from build123d import *

# Parameters (mm, degrees)
ESQUISSE1_W             = 34
ESQUISSE1_H             = 100.65
BOSS_EXTRU_1_DEPTH      = 12.5
ESQUISSE2_W             = 31
ESQUISSE2_H             = 97.65
ENL_V_MAT_EXTRU_1_DEPTH = 11
ESQUISSE5_R             = 2
BOSS_EXTRU_4_DEPTH      = 3
CONG_2_R                = 2
CONG_3_R                = 2
CONG_4_R                = 2
ESQUISSE7_W             = 7.5
ESQUISSE7_H             = 80
BOSS_EXTRU_6_DEPTH      = 1
ESQUISSE9_W             = 9.45
ESQUISSE9_H             = 80
BOSS_EXTRU_7_DEPTH      = 1.7
ESQUISSE11_W            = 15.5
ESQUISSE11_H            = 4.6
ENL_V_MAT_EXTRU_3_DEPTH = 3
CONG_7_R                = 1
ESQUISSE12_R            = 1.3
ENL_V_MAT_EXTRU_5_DEPTH = 3


with BuildPart() as part:
    # Esquisse1 → Boss.-Extru.1 (new body)
    with BuildSketch(Plane.XY):
        with Locations((17, 50.325)):
            Rectangle(ESQUISSE1_W, ESQUISSE1_H)
    extrude(amount=BOSS_EXTRU_1_DEPTH)

    # Esquisse2 → Enlèv. mat.-Extru.1 (cut)
    with BuildSketch(Plane.XY.offset(12.5)):
        with Locations((17, 50.325)):
            Rectangle(ESQUISSE2_W, ESQUISSE2_H)
    extrude(amount=-ENL_V_MAT_EXTRU_1_DEPTH, mode=Mode.SUBTRACT)

    # Esquisse5 → Boss.-Extru.4 (add)
    with BuildSketch(Plane.XY.offset(1.5)):
        with Locations((5.5, 63.5)):
            Circle(ESQUISSE5_R)
        with Locations((28.5, 63.5)):
            Circle(ESQUISSE5_R)
        with Locations((5.5, 5.5)):
            Circle(ESQUISSE5_R)
        with Locations((28.5, 5.5)):
            Circle(ESQUISSE5_R)
    extrude(amount=BOSS_EXTRU_4_DEPTH)

    # Congé2
    cong_2_edges = [part.edges().sort_by_distance(p)[0] for p in [
        (34, 0, 6.25),
    ]]
    fillet(cong_2_edges, radius=CONG_2_R)

    # Congé3
    cong_3_edges = [part.edges().sort_by_distance(p)[0] for p in [
        (34, 100.65, 6.25),
    ]]
    fillet(cong_3_edges, radius=CONG_3_R)

    # Congé4
    cong_4_edges = [part.edges().sort_by_distance(p)[0] for p in [
        (34, 50.325, 0),
        (33.414213562, 0.585786438, 0),
        (16, 100.65, 0),
        (33.414213562, 100.064213562, 0),
        (16, 0, 0),
    ]]
    fillet(cong_4_edges, radius=CONG_4_R)

    # Esquisse7 → Boss.-Extru.6 (add)
    with BuildSketch(Plane.ZY):
        with Locations((7, 55.45)):
            Rectangle(ESQUISSE7_W, ESQUISSE7_H)
    extrude(amount=BOSS_EXTRU_6_DEPTH)

    # Esquisse9 → Boss.-Extru.7 (add)
    with BuildSketch(Plane.ZY.offset(1)):
        with Locations((6.725, 55.45)):
            Rectangle(ESQUISSE9_W, ESQUISSE9_H)
    extrude(amount=BOSS_EXTRU_7_DEPTH)

    # Esquisse11 → Enlèv. mat.-Extru.3 (cut)
    with BuildSketch(Plane(origin=(0, 1.5, 0), x_dir=(1, 0, 0), z_dir=(0, 1, 0))):
        with Locations((14.724178104, -7.8)):
            Rectangle(ESQUISSE11_W, ESQUISSE11_H)
    extrude(amount=-ENL_V_MAT_EXTRU_3_DEPTH, mode=Mode.SUBTRACT)

    # Congé7
    cong_7_edges = [part.edges().sort_by_distance(p)[0] for p in [
        (-2.7, 55.45, 2),
        (-2.7, 15.45, 6.725),
        (-2.7, 55.45, 11.45),
        (-2.7, 95.45, 6.725),
    ]]
    fillet(cong_7_edges, radius=CONG_7_R)

    # Esquisse12 → Enlèv. mat.-Extru.5 (cut)
    with BuildSketch(Plane.XY.offset(4.5)):
        with Locations((5.5, 63.5)):
            Circle(ESQUISSE12_R)
        with Locations((28.5, 63.5)):
            Circle(ESQUISSE12_R)
        with Locations((5.5, 5.5)):
            Circle(ESQUISSE12_R)
        with Locations((28.5, 5.5)):
            Circle(ESQUISSE12_R)
    extrude(amount=-ENL_V_MAT_EXTRU_5_DEPTH, mode=Mode.SUBTRACT)


solid = part.part
Geometry check sheet. Reference: the model listing, model coordinates, mm. A direction names the side the tool comes from. Give positions to 0.01 mm unless a question says otherwise; leave off trailing zeros. Write each loop counter-clockwise with the first axis right and the second up, starting at its lowest first coordinate (ties: lowest second). Pieces come first, ordered by that corner, then holes. Notation, with made-up numbers: (65.5, 87.5) - (99.5, 87.5) arc R27 cw to (99.5, 110.5) - close; hole circle Ø3 at (-36, 52.25). An arc over 180 degrees is marked (long way). Put each result on its own line as item: value.
1. Set-up check for faces 1 (the flat face through (-1, 95.45, 7)), 2 (the flat face through (34, 50, 7)), 3 (the flat face through (5, 6, 1.5)): record each of +Z, -Z, +X, -X, +Y, -Y from which the full face is reachable in a straight line by a thin tool's end or side.
Ans:
face 1: +Z, -Z, -X, +Y
face 2: +Z, -Z, +X, +Y, -Y
face 3: +Z
2. Sectioned sample at A-A, the plane x = 15.5. Enter the section's corners in (y, z), plus the area to 3 significant figures.
Ans:
outline: (0, 2) arc R2 ccw to (2, 0) - (98.65, 0) arc R2 ccw to (100.65, 2) - (100.65, 12.5) - (99.15, 12.5) - (99.15, 1.5) - (1.5, 1.5) - (1.5, 5.5) - (0, 5.5) - close; (0, 10.1) - (1.5, 10.1) - (1.5, 12.5) - (0, 12.5) - close
area: 175 mm²
3. Draft check along Y on faces 4 (the flat face through (16, 0, 5)), 5 (the cylindrical face through (33.4, 51, 0.57)), 6 (the flat face through (1.5, 50, 7)). Enter one of: +Y half, -Y half, draft (parallel to the pull), parting line (faces both ways), or undercut.
Ans:
face 4: -Y half
face 5: draft
face 6: undercut
4. Sectioned sample at D-D, the plane x = 5.5. Enter the section's corners in (y, z).
Ans:
outline: (0, 2) arc R2 ccw to (2, 0) - (98.65, 0) arc R2 ccw to (100.65, 2) - (100.65, 12.5) - (99.15, 12.5) - (99.15, 1.5) - (65.5, 1.5) - (65.5, 4.5) - (64.8, 4.5) - (64.8, 1.5) - (62.2, 1.5) - (62.2, 4.5) - (61.5, 4.5) - (61.5, 1.5) - (7.5, 1.5) - (7.5, 4.5) - (6.8, 4.5) - (6.8, 1.5) - (4.2, 1.5) - (4.2, 4.5) - (3.5, 4.5) - (3.5, 1.5) - (1.5, 1.5) - (1.5, 12.5) - (0, 12.5) - close
5. Sectioned sample at C-C, the plane z = 8. Enter the section's corners in (x, y), plus the area to 3 significant figures.
Ans:
outline: (-2.7, 16.45) arc R1 ccw to (-1.7, 15.45) - (0, 15.45) - (0, 0) - (6.97, 0) - (6.97, 1.5) - (1.5, 1.5) - (1.5, 99.15) - (32.5, 99.15) - (32.5, 1.5) - (22.47, 1.5) - (22.47, 0) - (32, 0) arc R2 ccw to (34, 2) - (34, 98.65) arc R2 ccw to (32, 100.65) - (0, 100.65) - (0, 95.45) - (-1.7, 95.45) arc R1 ccw to (-2.7, 94.45) - close
area: 586 mm²
6. Sectioned sample at B-B, the plane y = 5.5. Enter the section's corners in (x, z), plus the area to 3 significant figures.
Ans:
outline: (0, 0) - (32, 0) arc R2 ccw to (34, 2) - (34, 12.5) - (32.5, 12.5) - (32.5, 1.5) - (30.5, 1.5) - (30.5, 4.5) - (29.8, 4.5) - (29.8, 1.5) - (27.2, 1.5) - (27.2, 4.5) - (26.5, 4.5) - (26.5, 1.5) - (7.5, 1.5) - (7.5, 4.5) - (6.8, 4.5) - (6.8, 1.5) - (4.2, 1.5) - (4.2, 4.5) - (3.5, 4.5) - (3.5, 1.5) - (1.5, 1.5) - (1.5, 12.5) - (0, 12.5) - close
area: 91.5 mm²
7. Thickness scan on line 1 (Y direction, x = 5.5, z = 3); line 2 (Y direction, x = 17.5, z = 4); line 3 (Y direction, x = 5, z = 3). Record the ranges inside material, lowest first.
Ans:
line 1: y = 0 to 1.5, 3.5 to 4.2, 6.8 to 7.5, 61.5 to 62.2, 64.8 to 65.5, 99.15 to 100.65
line 2: y = 0 to 1.5, 99.15 to 100.65
line 3: y = 0 to 1.5, 3.56 to 4.3, 6.7 to 7.44, 61.56 to 62.3, 64.7 to 65.44, 99.15 to 100.65
8. Go/stop test with flat-tipped pins: pin 1 (2 mm diameter, centred on x = 28.5, y = 63.5, fed in from +Z); pin 2 (0.8 mm diameter, centred on x = -0.5, y = 37, fed in from +Z); pin 3 (1.2 mm diameter, centred on x = 4.5, y = 6, fed in from +Z). Record where each tip stops, or that it passes through.
Ans:
pin 1: stops at z = 1.5
pin 2: stops at z = 10.75
pin 3: stops at z = 4.5
